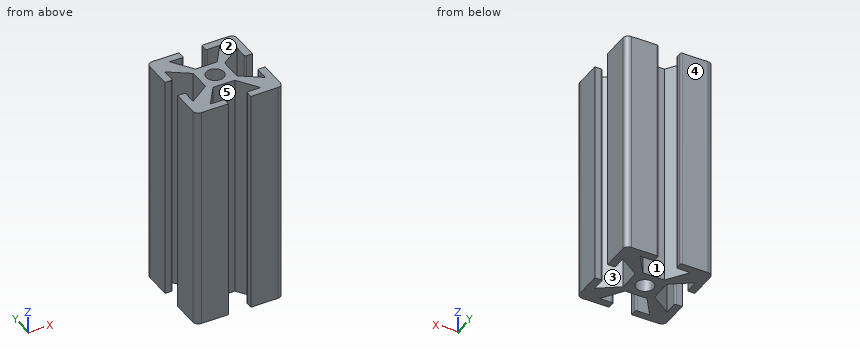
from build123d import *

# Parameters (mm, degrees)
SKETCH1_W                   = 25.4
SKETCH1_H                   = 25.4
BOSS_EXTRUDE1_DEPTH         = 65.786
FILLET1_R                   = 1.5875
HOLE1_OUTLINE_R             = 2.5527
HOLE1_DEPTH                 = 65.786
SKETCH7_W                   = 6.5278
SKETCH7_H                   = 2.2352
CUT_EXTRUDE2_DEPTH          = 65.786
FILLET4_R                   = 0.396875
CIRPATTERN2_DEPTH           = 65.786
F_1_4_20_TAPPED_HOLE1_D     = 5.1054
F_1_4_20_TAPPED_HOLE1_DEPTH = 6.35
F_1_4_20_TAPPED_HOLE1_TIP   = 1.533816902


# Read off the part's stored shape, not the designer's step: Hole1, CirPattern2
with BuildPart() as part:
    # Sketch1 → Boss-Extrude1 (new body)
    with BuildSketch(Plane.XY):
        Rectangle(SKETCH1_W, SKETCH1_H)
    extrude(amount=BOSS_EXTRUDE1_DEPTH)

    # Fillet1
    fillet1_edges = [part.edges().sort_by_distance(p)[0] for p in [
        (12.7, -12.7, 32.893),
        (-12.7, -12.7, 32.893),
        (-12.7, 12.7, 32.893),
        (12.7, 12.7, 32.893),
    ]]
    fillet(fillet1_edges, radius=FILLET1_R)

    # Hole1 outline → Hole1 (cut)
    with BuildSketch(Plane.XY):
        with Locations((0, -0.048792482)):
            Circle(HOLE1_OUTLINE_R)
    extrude(amount=HOLE1_DEPTH, mode=Mode.SUBTRACT)

    # Sketch7 → Cut-Extrude2 (cut)
    with BuildSketch(Plane.XY.offset(65.786)):
        with Locations((0, 11.5824)):
            Rectangle(SKETCH7_W, SKETCH7_H)
        Polygon((-3.175, 4.5212), (-7.3025, 10.4648), (7.3025, 10.4648), (3.175, 4.5212), align=None)
    extrude(amount=-CUT_EXTRUDE2_DEPTH, mode=Mode.SUBTRACT)

    # Fillet4
    fillet4_edges = [part.edges().sort_by_distance(p)[0] for p in [
        (-3.2639, 10.4648, 32.893),
        (-3.2639, 12.7, 32.893),
        (3.2639, 12.7, 32.893),
        (3.2639, 10.4648, 32.893),
    ]]
    fillet(fillet4_edges, radius=FILLET4_R)

    # CirPattern2 outline → CirPattern2 (cut)
    with BuildSketch(Plane.XY):
        with BuildLine():
            ThreePointArc((-3.660775, -10.562384964), (-3.380141996, -10.67862696), (-3.2639, -10.959259964))
            Line((-3.2639, -10.959259964), (-3.2639, -12.7))
            Line((-3.2639, -12.7), (3.2639, -12.7))
            Line((3.2639, -12.7), (3.2639, -10.959259964))
            ThreePointArc((3.2639, -10.959259964), (3.380141996, -10.67862696), (3.660775, -10.562384964))
            Line((3.660775, -10.562384964), (7.3025, -10.562384964))
            Line((7.3025, -10.562384964), (3.175, -4.618784964))
            Line((3.175, -4.618784964), (-3.175, -4.618784964))
            Line((-3.175, -4.618784964), (-7.3025, -10.562384964))
            Line((-7.3025, -10.562384964), (-3.660775, -10.562384964))
        make_face()
        with BuildLine():
            Line((-12.7, -3.312692482), (-10.910467482, -3.312692482))
            ThreePointArc((-10.910467482, -3.312692482), (-10.629834478, -3.428934478), (-10.513592482, -3.709567482))
            Line((-10.513592482, -3.709567482), (-10.513592482, -7.351292482))
            Line((-10.513592482, -7.351292482), (-4.569992482, -3.223792482))
            Line((-4.569992482, -3.223792482), (-4.569992482, 3.126207518))
            Line((-4.569992482, 3.126207518), (-10.513592482, 7.253707518))
            Line((-10.513592482, 7.253707518), (-10.513592482, 3.611982518))
            ThreePointArc((-10.513592482, 3.611982518), (-10.629834478, 3.331349514), (-10.910467482, 3.215107518))
            Line((-10.910467482, 3.215107518), (-12.7, 3.215107518))
            Line((-12.7, 3.215107518), (-12.7, -3.312692482))
        make_face()
        with BuildLine():
            ThreePointArc((10.513592482, -3.709567482), (10.629834478, -3.428934478), (10.910467482, -3.312692482))
            Line((10.910467482, -3.312692482), (12.7, -3.312692482))
            Line((12.7, -3.312692482), (12.7, 3.215107518))
            Line((12.7, 3.215107518), (10.910467482, 3.215107518))
            ThreePointArc((10.910467482, 3.215107518), (10.629834478, 3.331349514), (10.513592482, 3.611982518))
            Line((10.513592482, 3.611982518), (10.513592482, 7.253707518))
            Line((10.513592482, 7.253707518), (4.569992482, 3.126207518))
            Line((4.569992482, 3.126207518), (4.569992482, -3.223792482))
            Line((4.569992482, -3.223792482), (10.513592482, -7.351292482))
            Line((10.513592482, -7.351292482), (10.513592482, -3.709567482))
        make_face()
    extrude(amount=CIRPATTERN2_DEPTH, mode=Mode.SUBTRACT)

    # 1/4-20 Tapped Hole1
    with Locations(Plane(origin=(0, -0.048792482, 65.786), x_dir=(1, 0, 0), z_dir=(0, 0, 1))):
        with Locations((0, 0)):
            Hole(F_1_4_20_TAPPED_HOLE1_D / 2, depth=F_1_4_20_TAPPED_HOLE1_DEPTH)
            with Locations((0, 0, -(F_1_4_20_TAPPED_HOLE1_DEPTH + F_1_4_20_TAPPED_HOLE1_TIP / 2))):  # 118° drill point
                Cone(0, F_1_4_20_TAPPED_HOLE1_D / 2, F_1_4_20_TAPPED_HOLE1_TIP, mode=Mode.SUBTRACT)


solid = part.part
Can you work these out from the model? Positions are in its coordinate system, mm. Face numbers are marked on the shaded views. A direction names the side the tool comes from. Coordinates: 2 decimals unless noted, no trailing zeros. Order: outer loops, then holes, each group sorted by start corner. A loop starts at its lowest first (then second) coordinate and runs counter-clockwise, first axis right, second up. Notation, with made-up numbers: (84.25, 24) -> (130.25, 24) arc R9 cw to (130.25, 29) -> close; hole circle Ø5 at (-36.75, -32). An arc over 180 degrees is marked (long way). Use one line per item in the form item = value.
Q1. Which directions (+Z, -Z, +X, -X, +Y, -Y) give clear straight access to the entire face, cutting with the end or side of a thin tool? Please do the marked faces 3, 4 and 5.
From the geometry:
face_3 = +Z, -Z
face_4 = +Z, -Z, +X, -X, +Y
face_5 = +Z, -Z, -Y
Q2. Imagine slicing it at B-B, the plane y = -9.75. List the corners of the cut face in (x, z) for me, then the cut area to 3 significant figures.
From the geometry:
outline = (-12.7, 0) -> (-6.74, 0) -> (-6.74, 65.79) -> (-12.7, 65.79) -> close; (6.74, 0) -> (12.7, 0) -> (12.7, 65.79) -> (6.74, 65.79) -> close
area = 784 mm²
Q3. Imagine slicing it at C-C, the plane y = 5.25. List the corners of the cut face in (x, z) for me, then the cut area to 3 significant figures.
From the geometry:
outline = (-12.7, 0) -> (-10.51, 0) -> (-10.51, 65.79) -> (-12.7, 65.79) -> close; (-7.63, 0) -> (-3.68, 0) -> (-3.68, 65.79) -> (-7.63, 65.79) -> close; (3.68, 0) -> (7.63, 0) -> (7.63, 65.79) -> (3.68, 65.79) -> close; (10.51, 0) -> (12.7, 0) -> (12.7, 65.79) -> (10.51, 65.79) -> close
area = 807 mm²
Q4. Will these pins go through, and if not, where does the flat tip stop? P1, Ø1, axis at y = 2, z = 39.5, coming from the -X side; P2, Ø1.4, axis at y = -12, z = 46, coming from the +X side; P3, Ø1.4, axis at x = -12, z = 38, coming from the +Y side; P4, Ø3, axis at x = 0, y = -0.05, coming from the +Z side.
From the geometry:
P1 = -4.57
P2 = 12.69
P3 = 12.69
P4 = through
Q5. Imagine slicing it at A-A, the plane x = 0. List the corners of the cut face in (y, z) for me, then the cut area to 3 significant figures.
From the geometry:
outline = (-4.62, 0) -> (-2.6, 0) -> (-2.6, 65.79) -> (-4.62, 65.79) -> close; (2.5, 0) -> (4.52, 0) -> (4.52, 65.79) -> (2.5, 65.79) -> close
area = 265 mm²
Q6. I need wall thicknesses on L1, parallel to Y at x = -11.25, z = 55; L2, parallel to X at y = 6.5, z = 3; L3, parallel to X at y = 6.75, z = 40. Which ranges of each line are inside material? Lowest first, please.
From the geometry:
L1 = -12.69 to -3.31, 3.22 to 12.69
L2 = -12.7 to -10.51, -9.43 to -4.55, 4.55 to 9.43, 10.51 to 12.7
L3 = -12.7 to -10.51, -9.79 to -4.72, 4.72 to 9.79, 10.51 to 12.7
Q7. We'd pull the mould along X, two halves only. Please class the marked faces 1 and 2: released by +X, released by -X, zero draft, split by the parting line, or undercut.
From the geometry:
face_1 = undercut
face_2 = zero draft
